Here's how the part is built. I have some questions about the finished solid (model axes, mm). A direction names the side the tool comes from. Coordinates: 2 decimals unless noted, no trailing zeros. Loops run counter-clockwise (first coordinate to the right, second up) from the corner with the lowest first, then second, coordinate; pieces in that order, holes last. Notation, with made-up numbers: (84, 0) -> (103, 0) arc R24 ccw to (103, 35) -> close; hole circle Ø7 at (81, 75.5). An arc over 180 degrees is marked (long way). Answer as a JSON object with one key per item and string values. Group by question number.
Q1. Thinking about a two-plate mould opening in Z: for faces 6 (the cylindrical face through (24.614, -39.86, 58.872)), 7 (the flat face through (30, -5, 20)), 8 (the flat face through (34, -2, 30)), which applies, released by +Z, released by -Z, zero draft, split by the parting line, or undercut?
Q2. I'm going to push flat-ended pins straight in: pin 1 (8 mm diameter, centred on x = 7, y = -37, fed in from +Z); pin 2 (5 mm diameter, centred on y = -40.5, z = 24.5, fed in from -X); pin 3 (8 mm diameter, centred on y = -25.5, z = 19.5, fed in from -X). Where does each tip first touch, or does it pass through?
Q3. I want a section at A-A on x = -12. Write out the boundary of the cut face in (y, z).
Q4. I need wall thicknesses on line 1 (Z direction, x = 20, y = -44.5); line 2 (Y direction, x = -10, z = 7.75); line 3 (Z direction, x = 3, y = 33). Which ranges of each line are inside material? Lowest first, please.
Q5. I want a section at D-D on x = 24. Write out the boundary of the cut face in (y, z), then the cut area to 3 significant figures.
Q6. I want a section at C-C on z = 42.5. Write out the boundary of the cut face in (x, y), then the cut area to 3 significant figures.
Q7. On a 3-axis mill with a long thin cutter (end or side, diameter ignored), from which of +Z, -Z, +X, -X, +Y, -Y can I reach the whole of each face in a straight line? I mean faces 1 (the cylindrical face through (21.445, 20.979, 19.86)), 2 (the flat face through (-30, -35, 8)), 3 (the flat face through (12, -50, 27)), 4 (the flat face through (0, 31, 11)), 5 (the flat face through (-20, -40, 25)). Say none if no direction works.
Q8. I want a section at B-B on y = -3. Write out the boundary of the cut face in (x, z) (3 decimals).
```python
from build123d import *

# Parameters (mm, degrees)
BOSS_EXTRUDE1_DEPTH = 30
SKETCH2_R           = 10
BOSS_EXTRUDE2_DEPTH = 10
SKETCH3_W           = 70
SKETCH3_H           = 20
BOSS_EXTRUDE3_DEPTH = 70
CUT_EXTRUDE1_DEPTH  = 50
SKETCH6_R           = 10
CUT_EXTRUDE2_DEPTH  = 50


with BuildPart() as part:
    # Sketch1 → Boss-Extrude1 (new body)
    with BuildSketch(Plane.XY):
        with BuildLine():
            Line((0, 30), (0, 40))
            ThreePointArc((0, 40), (28.284271247, 28.284271247), (40, 0))
            Line((40, 0), (40, -30))
            Line((40, -30), (10, -30))
            Line((10, -30), (10, -20))
            Line((10, -20), (20, -10))
            Line((20, -10), (30, -10))
            Line((30, -10), (30, 0))
            ThreePointArc((30, 0), (21.213203436, 21.213203436), (0, 30))
        make_face()
    extrude(amount=BOSS_EXTRUDE1_DEPTH)

    # Sketch2 → Boss-Extrude2 (add)
    with BuildSketch(Plane.XY):
        with BuildLine():
            Line((0, 40), (0, 10))
            Line((0, 10), (-10, 10))
            ThreePointArc((-10, 10), (-24.142135624, 4.142135624), (-30, -10))
            Line((-30, -10), (-30, -50))
            Line((-30, -50), (40, -50))
            Line((40, -50), (40, 0))
            ThreePointArc((40, 0), (28.284271247, 28.284271247), (0, 40))
        make_face()
        with Locations((-10, -10)):
            Circle(SKETCH2_R, mode=Mode.SUBTRACT)
    extrude(amount=BOSS_EXTRUDE2_DEPTH)

    # Sketch3 → Boss-Extrude3 (add)
    with BuildSketch(Plane.XY.offset(10)):
        with Locations((5, -40)):
            Rectangle(SKETCH3_W, SKETCH3_H)
    extrude(amount=BOSS_EXTRUDE3_DEPTH)

    # Sketch4 → Cut-Extrude1 (cut)
    with BuildSketch(Plane(origin=(0, -30, 0), x_dir=(1, 0, 0), z_dir=(0, 1, 0))):
        with BuildLine():
            Line((-20, -30), (-20, -20))
            Line((-20, -20), (-30, -20))
            Line((-30, -20), (-30, -80))
            Line((-30, -80), (40, -80))
            Line((40, -80), (40, -50))
            ThreePointArc((40, -50), (20, -70), (0, -50))
            ThreePointArc((0, -50), (-5.857864376, -35.857864376), (-20, -30))
        make_face()
    extrude(amount=-CUT_EXTRUDE1_DEPTH, mode=Mode.SUBTRACT)

    # Sketch6 → Cut-Extrude2 (cut)
    with BuildSketch(Plane(origin=(0, -30, 0), x_dir=(1, 0, 0), z_dir=(0, 1, 0))):
        with Locations((20, -50)):
            Circle(SKETCH6_R)
    extrude(amount=-CUT_EXTRUDE2_DEPTH, mode=Mode.SUBTRACT)


solid = part.part
```
Result set:
{
 "1": {"face 6": "undercut", "face 7": "zero draft", "face 8": "released by +Z"},
 "2": {"pin 1": "stops at z = 67.86", "pin 2": "stops at x = -20", "pin 3": "stops at x = 10"},
 "3": {"outline": "(-50, 0) -> (-19.8, 0) -> (-19.8, 10) -> (-30, 10) -> (-30, 31.67) -> (-50, 31.67) -> close; (-0.2, 0) -> (9.9, 0) -> (9.9, 10) -> (-0.2, 10) -> close"},
 "4": {"line 1": "z = 0 to 40, 60 to 70", "line 2": "y = -50 to -20, 0 to 10", "line 3": "z = 0 to 30"},
 "5": {"outline": "(-50, 0) -> (32, 0) -> (32, 30) -> (18, 30) -> (18, 10) -> (-10, 10) -> (-10, 30) -> (-30, 30) -> (-30, 40.83) -> (-50, 40.83) -> close; (-50, 59.17) -> (-30, 59.17) -> (-30, 69.6) -> (-50, 69.6) -> close", "area": "2,330 mm²"},
 "6": {"outline": "(-1.46, -50) -> (13.39, -50) -> (13.39, -30) -> (-1.46, -30) -> close; (26.61, -50) -> (40, -50) -> (40, -30) -> (26.61, -30) -> close", "area": "565 mm²"},
 "7": {"face 1": "+Z, -X", "face 2": "+Z, -Z, -X, +Y, -Y", "face 3": "+Z, -Z, +X, -X, -Y", "face 4": "+Z, -Z, -X, +Y", "face 5": "+Z, -X, +Y, -Y"},
 "8": {"outline": "(-28.735, 0) -> (-17.141, 0) -> (-17.141, 10) -> (-28.735, 10) -> close; (-2.859, 0) -> (40, 0) -> (40, 30) -> (30, 30) -> (30, 10) -> (-2.859, 10) -> close"}
}
